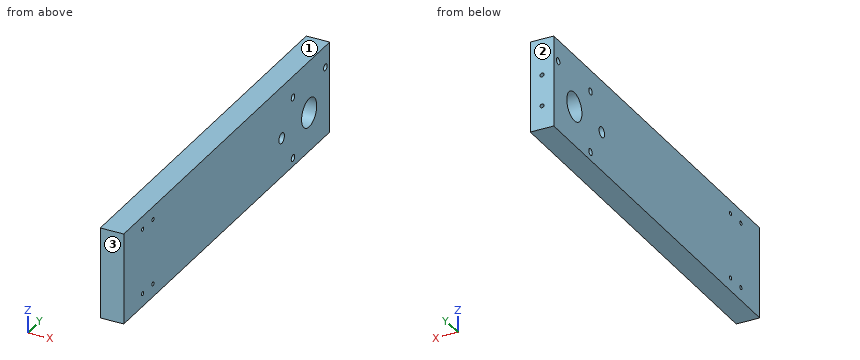
```python
from build123d import *

# Parameters (mm, degrees)
CROQUIS2_W              = 70
CROQUIS2_H              = 300
CROQUIS2_R              = 1.5
CROQUIS2_R_2            = 4
CROQUIS2_R_3            = 2.5
CROQUIS2_R_4            = 11
SALIENTE_EXTRUIR1_DEPTH = 18
CROQUIS3_R              = 1.5
CORTAR_EXTRUIR1_DEPTH   = 14


with BuildPart() as part:
    # Croquis2 → Saliente-Extruir1 (new body)
    with BuildSketch(Plane(origin=(0, 0, 0), x_dir=(0, 0, -1), z_dir=(1, 0, 0))):
        Rectangle(CROQUIS2_W, CROQUIS2_H)
        with Locations((25, -122.5)):
            Circle(CROQUIS2_R, mode=Mode.SUBTRACT)
        with Locations((-25, -122.5)):
            Circle(CROQUIS2_R, mode=Mode.SUBTRACT)
        with Locations((25, -107.5)):
            Circle(CROQUIS2_R, mode=Mode.SUBTRACT)
        with Locations((-25, -107.5)):
            Circle(CROQUIS2_R, mode=Mode.SUBTRACT)
        with Locations((5, 80)):
            Circle(CROQUIS2_R_2, mode=Mode.SUBTRACT)
        with Locations((28.57, 96.43)):
            Circle(CROQUIS2_R_3, mode=Mode.SUBTRACT)
        with Locations((5, 120)):
            Circle(CROQUIS2_R_4, mode=Mode.SUBTRACT)
        with Locations((-18.57, 96.43)):
            Circle(CROQUIS2_R_3, mode=Mode.SUBTRACT)
        with Locations((-18.57, 143.57)):
            Circle(CROQUIS2_R_3, mode=Mode.SUBTRACT)
    extrude(amount=SALIENTE_EXTRUIR1_DEPTH)

    # Croquis3 → Cortar-Extruir1 (cut)
    with BuildSketch(Plane(origin=(0, 150, 0), x_dir=(1, 0, 0), z_dir=(0, 1, 0))):
        with Locations((9, -7)):
            Circle(CROQUIS3_R)
        with Locations((9, 17)):
            Circle(CROQUIS3_R)
    extrude(amount=-CORTAR_EXTRUIR1_DEPTH, mode=Mode.SUBTRACT)


solid = part.part
```
CAD build for the part. Positions are in the model's coordinates, mm. Face numbers are marked on the shaded views. Coordinates: 2 decimals unless noted, no trailing zeros. Write each loop counter-clockwise with the first axis right and the second up, starting at its lowest first coordinate (ties: lowest second). Pieces come first, ordered by that corner, then holes.
(1) Two-plate mould, pull along Y, no slides. Class the marked faces 1, 2 and 3: +Y half, -Y half, draft (parallel to the pull), parting line (faces both ways), or undercut.
(2) Cut at C-C, the plane z = 3. List the corners of the cut face in (x, y), and give its area (3 significant figures).
(3) Cut at B-B, the plane x = 14. Count the separate pieces of the cut face and the enclosed holes in it, and give its area (3 significant figures).
(4) Cut at A-A, the plane y = 143.57. List the corners of the cut face in (x, z).
(5) Drill centre lines: probe 1 along Y at (x, z) = (11, -5); probe 2 along Z at (x, y) = (9, 139.5); probe 3 along Y at (x, z) = (13.75, 25). Where is each one in solid material? Low to high.
(6) Flat gauge pin, fed straight in: pin 1 (0.9 mm diameter, centred on x = 9.5, z = -16.5, fed in from +Y). Where does the tip first touch, or does it go through?
Geometry says:
1. face 1: draft
1. face 2: +Y half
1. face 3: -Y half
2. outline: (0, -150) - (18, -150) - (18, 112.45) - (0, 112.45) - close; (0, 127.55) - (18, 127.55) - (18, 150) - (0, 150) - close
2. area: 5,130 mm2
3. separate pieces: 1
3. enclosed holes: 9
3. area: 20,500 mm2
4. outline: (0, -35) - (18, -35) - (18, 16.07) - (0, 16.07) - close; (0, 21.07) - (18, 21.07) - (18, 35) - (0, 35) - close; hole circle Ø3 at (9, -17); hole circle Ø3 at (9, 7)
5. probe 1: y = -150 to 76, 84 to 109, 131 to 150
5. probe 2: z = -35 to -18.5, -15.5 to 5.5, 8.5 to 35
5. probe 3: y = -150 to -124, -121 to -109, -106 to 150
6. pin 1: stops at y = 136
